For this review, take the finished solid that the model builds, in its own axes (mm). Face numbers are marked on the shaded views. A direction names the side the tool comes from. Round coordinates to 2 decimals unless told otherwise and drop trailing zeros. Loops run counter-clockwise (first coordinate to the right, second up) from the corner with the lowest first, then second, coordinate; pieces in that order, holes last.
1. Tool access review of the marked faces 1 and 2: name each direction out of +Z, -Z, +X, -X, +Y, -Y from which nothing blocks a thin tool from reaching the whole face with its end or side.
2. Consider section D-D on x = -8.15. State the section outline as (y, z) points.
3. Clearance check with flat-ended pins moving along their axes: pin 1 Ø2 at (y, z) = (4.5, 3.5) entering from +X; pin 2 Ø0.8 at (y, z) = (4, -2) entering from +X; pin 3 Ø1.1 at (x, z) = (-4.5, -2) entering from -Y. State where each tip first meets the part, or that it passes through.
4. To check wall thickness, follow line 1 along Z through (x, y) = (-7.95, 4.6); line 2 along Z through (x, y) = (-5.95, 4.6); line 3 along Y through (x, z) = (-6.05, 6). State the ranges of each line that lie inside material, in increasing order.
5. Consider section A-A on y = 4.05. State the section outline as (x, z) points.
6. Consider section C-C on z = -1. State the section outline as (x, y) points.
7. Consider section B-B on x = -5.05. State the section outline as (y, z) points.
from build123d import *

# Parameters (mm, degrees)
SKETCH_1_R          = 1.5
EXTRUDE_1_DEPTH     = 9
SKETCH_2_R          = 3
EXTRUDE_2_DEPTH     = 2.5
CUT_EXTRUDE_3_DEPTH = 1


with BuildPart() as part:
    # 草图1 → 凸台-拉伸1 (new body)
    with BuildSketch(Plane.XY):
        with Locations((-5.944112119, 3.006217623)):
            Circle(SKETCH_1_R)
    extrude(amount=EXTRUDE_1_DEPTH)

    # 草图2 → 凸台-拉伸2 (add)
    with BuildSketch(Plane(origin=(0, 0, 0), x_dir=(-1, 0, 0), z_dir=(0, 0, -1))):
        with Locations((5.944112119, 3.006217623)):
            Circle(SKETCH_2_R)
    extrude(amount=EXTRUDE_2_DEPTH)

    # 草图4 → 切除-拉伸3 (cut)
    with BuildSketch(Plane(origin=(0, 0, -2.5), x_dir=(-1, 0, 0), z_dir=(0, 0, -1))):
        Polygon((3.944112119, 3.256217623), (5.694112119, 3.256217623), (5.694112119, 5.006217623), (6.194112119, 5.006217623), (6.194112119, 3.256217623), (7.944112119, 3.256217623), (7.944112119, 2.756217623), (6.194112119, 2.756217623), (6.194112119, 1.006217623), (5.694112119, 1.006217623), (5.694112119, 2.756217623), (3.944112119, 2.756217623), align=None)
    extrude(amount=-CUT_EXTRUDE_3_DEPTH, mode=Mode.SUBTRACT)


solid = part.part
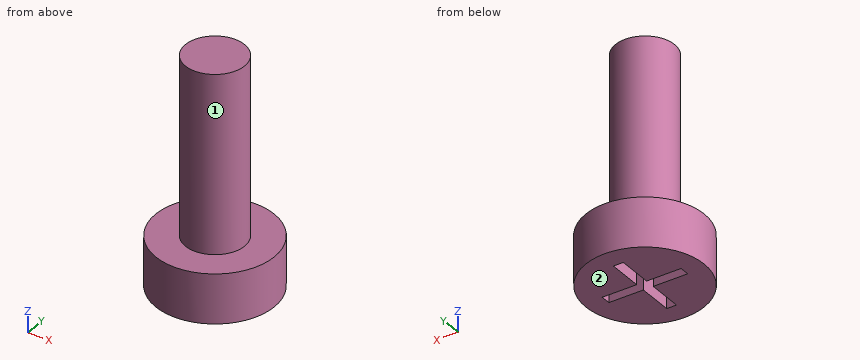
Resolved:
1. face 1: +Z
1. face 2: -Z, +X, -X, +Y, -Y
2. outline: (0.97, -2.5) - (5.04, -2.5) - (5.04, 0) - (0.97, 0) - close
3. pin 1: stops at x = -4.53
3. pin 2: stops at x = -3
3. pin 3: stops at y = 0.14
4. line 1: z = -2.5 to 0
4. line 2: z = -1.5 to 0
4. line 3: y = 1.51 to 4.5
5. outline: (-8.76, -2.5) - (-6.19, -2.5) - (-6.19, -1.5) - (-5.69, -1.5) - (-5.69, -2.5) - (-3.13, -2.5) - (-3.13, 0) - (-4.87, 0) - (-4.87, 9) - (-7.02, 9) - (-7.02, 0) - (-8.76, 0) - close
6. outline: circle Ø6 at (-5.94, 3.01)
7. outline: (0.14, -2.5) - (2.76, -2.5) - (2.76, -1.5) - (3.26, -1.5) - (3.26, -2.5) - (5.87, -2.5) - (5.87, 0) - (4.21, 0) - (4.21, 9) - (1.8, 9) - (1.8, 0) - (0.14, 0) - close
